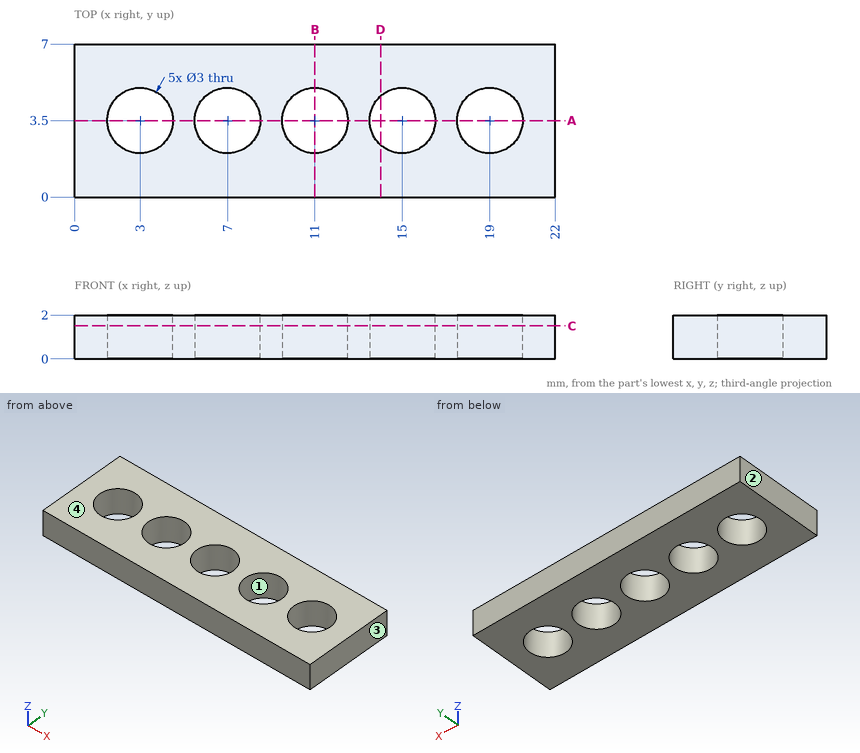
Geometry check sheet. Reference: drawing and pictorial views, mm from the part's lowest x, y, z. Give positions to 0.01 mm unless a question says otherwise; leave off trailing zeros. Order: outer loops, then holes, each group sorted by start corner. A loop starts at its lowest first (then second) coordinate and runs counter-clockwise, first axis right, second up. Notation, with made-up numbers: M -40,25.5 L -15,25.5 A7 cw -15,35.5 Z; hole C 64,-8 d9. An arc over 180 degrees is marked long. Answer as a JSON object with one key per item and string values. Group by question number.
1) Depth check by flat-ended pin: pin 1 Ø4 at (x, y) = (19, 3.5) entering from +Z. Enter the tip coordinate at first touch or a pass-through.
2) Cross-section at B-B (x = 11). Enter the section's corners in (y, z).
3) Scan lines: line 1 along X through (y, z) = (3.5, 0.5); line 2 along Y through (x, z) = (15, 0.9); line 3 along X through (y, z) = (4.75, 1.15). Record each from-to range of solid material in increasing order. Write a range as [from, to].
4) Mould release check, pull along X, two halves, no side actions. Record for the marked faces 1, 2, 3 and 4: released by +X, released by -X, zero draft, split by the parting line, or undercut.
5) Cross-section at A-A (y = 3.5). Enter the section's corners in (x, z).
6) Cross-section at D-D (x = 14). Enter the section's corners in (y, z).
7) Cross-section at C-C (z = 1.5). Enter the section's corners in (x, y), then the cut area to 3 significant figures.
Result sheet:
{
 "1": {"pin 1": "stops at z = 2"},
 "2": {"outline": "M 0,0 L 2,0 L 2,2 L 0,2 Z; M 5,0 L 7,0 L 7,2 L 5,2 Z"},
 "3": {"line 1": "x = [0, 1.5], [4.5, 5.5], [8.5, 9.5], [12.5, 13.5], [16.5, 17.5], [20.5, 22]", "line 2": "y = [0, 2], [5, 7]", "line 3": "x = [0, 2.17], [3.83, 6.17], [7.83, 10.17], [11.83, 14.17], [15.83, 18.17], [19.83, 22]"},
 "4": {"face 1": "undercut", "face 2": "released by -X", "face 3": "released by +X", "face 4": "zero draft"},
 "5": {"outline": "M 0,0 L 1.5,0 L 1.5,2 L 0,2 Z; M 4.5,0 L 5.5,0 L 5.5,2 L 4.5,2 Z; M 8.5,0 L 9.5,0 L 9.5,2 L 8.5,2 Z; M 12.5,0 L 13.5,0 L 13.5,2 L 12.5,2 Z; M 16.5,0 L 17.5,0 L 17.5,2 L 16.5,2 Z; M 20.5,0 L 22,0 L 22,2 L 20.5,2 Z"},
 "6": {"outline": "M 0,0 L 2.38,0 L 2.38,2 L 0,2 Z; M 4.62,0 L 7,0 L 7,2 L 4.62,2 Z"},
 "7": {"outline": "M 0,0 L 22,0 L 22,7 L 0,7 Z; hole C 3,3.5 d3; hole C 7,3.5 d3; hole C 11,3.5 d3; hole C 15,3.5 d3; hole C 19,3.5 d3", "area": "119 mm2"}
}
